from build123d import *

# Parameters (mm, degrees)
SKETCH1_R                               = 32
SKETCH1_R_2                             = 20
BOSS_EXTRUDE1_DEPTH                     = 6
SKETCH1_2_R                             = 20
BOSS_EXTRUDE2_DEPTH                     = 60
CBORE_FOR_M6_HEX_HEAD_BOLT1_D           = 30
CBORE_FOR_M6_HEX_HEAD_BOLT1_CBORE_D     = 40
CBORE_FOR_M6_HEX_HEAD_BOLT1_CBORE_DEPTH = 2.3
SKETCH7_R                               = 3.25
CUT_EXTRUDE1_DEPTH                      = 6
CHAMFER1_SIZE                           = 0.5


with BuildPart() as part:
    # Sketch1 → Boss-Extrude1 (new body)
    with BuildSketch(Plane.XY):
        Circle(SKETCH1_R)
        Circle(SKETCH1_R_2, mode=Mode.SUBTRACT)
    extrude(amount=BOSS_EXTRUDE1_DEPTH)

    # Sketch1<2> → Boss-Extrude2 (add)
    with BuildSketch(Plane.XY):
        Circle(SKETCH1_2_R)
    extrude(amount=BOSS_EXTRUDE2_DEPTH)

    # CBORE for M6 Hex Head Bolt1 (through all)
    with Locations(Plane(origin=(0, 0, 0), x_dir=(-1, 0, 0), z_dir=(0, 0, -1))):
        with Locations((0, 0)):
            CounterBoreHole(CBORE_FOR_M6_HEX_HEAD_BOLT1_D / 2, CBORE_FOR_M6_HEX_HEAD_BOLT1_CBORE_D / 2, CBORE_FOR_M6_HEX_HEAD_BOLT1_CBORE_DEPTH)

    # Sketch7 → Cut-Extrude1 (cut)
    with BuildSketch(Plane(origin=(0, 0, 0), x_dir=(-1, 0, 0), z_dir=(0, 0, -1))):
        with Locations((0, 25)):
            Circle(SKETCH7_R)
        with Locations((25, 0)):
            Circle(SKETCH7_R)
        with Locations((0, -25)):
            Circle(SKETCH7_R)
        with Locations((-25, 0)):
            Circle(SKETCH7_R)
    extrude(amount=-CUT_EXTRUDE1_DEPTH, mode=Mode.SUBTRACT)

    # Chamfer1
    chamfer1_edges = [part.edges().sort_by_distance(p)[0] for p in [
        (20, 0, 0),
        (-15, 0, 60),
        (-32, 0, 0),
        (3.25, 25, 6),
        (3.25, 25, 0),
        (-21.75, 0, 6),
        (-21.75, 0, 0),
        (3.25, -25, 6),
        (3.25, -25, 0),
        (28.25, 0, 6),
        (28.25, 0, 0),
        (-32, 0, 6),
        (-20, 0, 6),
    ]]
    chamfer(chamfer1_edges, length=CHAMFER1_SIZE)


solid = part.part
Design review of the part built by this model. Coordinates are the model's own, in mm. Round coordinates to 2 decimals unless told otherwise and drop trailing zeros. Write each loop counter-clockwise with the first axis right and the second up, starting at its lowest first coordinate (ties: lowest second). Pieces come first, ordered by that corner, then holes. Notation, with made-up numbers: (86, 31) - (123, 31) arc R16 ccw to (123, 46) - close; hole circle Ø3 at (33.25, 65). An arc over 180 degrees is marked (long way). Return JSON: item names as keys, results as strings. Group by question number.
Item 1: We need section C-C on z = 20.5. Write out the cut boundary in (x, y).
Item 2: We need section A-A on y = 0. Give the number of separate pieces and of enclosed holes in the cut face, and give its area (3 significant figures).
Item 3: Insertion check: P1, Ø3, axis at x = -2, z = 33, coming from the +Y side; P2, Ø6, axis at x = 7, z = 15, coming from the -Y side; P3, Ø5, axis at x = -2.5, y = -25, coming from the +Z side. Each pin has a flat end and moves straight along its axis. Give the tip position at first contact, or say it passes through.
Item 4: For probe 1 along Y at (x, z) = (0, 3.3); probe 2 along Y at (x, z) = (0, 33); probe 3 along X at (y, z) = (-0.5, 37), list the stretches that pass through material, from the lowest coordinate up. Write a range as [from, to].
Item 5: The part is to be moulded in two halves that separate along X. For faces 1 (the face through (-6.94, -31.24, 2.96)), 2 (the face through (10.3, -11.8, 60)), 3 (the face through (-3, 15, 2.3)), say which applies: pulls with the +X half, pulls with the -X half, needs draft (parallel to the pull), parting line crosses it, or undercut.
Model answer:
{
 "1": {"outline": "circle Ø40 at (0, 0); hole circle Ø30 at (0, 0)"},
 "2": {"separate pieces": "4", "enclosed holes": "0", "area": "641 mm²"},
 "3": {"P1": "stops at y = 19.99", "P2": "stops at y = -19.6", "P3": "stops at z = 6"},
 "4": {"probe 1": "y = [-32, -28.25], [-21.75, -15], [15, 21.75], [28.25, 32]", "probe 2": "y = [-20, -15], [15, 20]", "probe 3": "x = [-19.99, -14.99], [14.99, 19.99]"},
 "5": {"face 1": "parting line crosses it", "face 2": "needs draft", "face 3": "undercut"}
}
